```python
from build123d import *

# Parameters (mm, degrees)
SKETCH1_W           = 140
SKETCH1_H           = 60
SKETCH1_R           = 2.0955
BOSS_EXTRUDE1_DEPTH = 6.35
SKETCH2_W           = 16
SKETCH2_H           = 10
SKETCH2_R           = 2
BOSS_EXTRUDE2_DEPTH = 6.35
FILLET1_R           = 2


with BuildPart() as part:
    # Sketch1 → Boss-Extrude1 (new body)
    with BuildSketch(Plane.XZ):
        with Locations((-8.25, 0)):
            Rectangle(SKETCH1_W, SKETCH1_H)
        with Locations(Location((-73.25, 25, 0), (0, 0, 270))):
            Circle(SKETCH1_R, mode=Mode.SUBTRACT)
        with Locations(Location((0, 25, 0), (0, 0, 270))):
            Circle(SKETCH1_R, mode=Mode.SUBTRACT)
        with Locations(Location((56.75, 25, 0), (0, 0, 270))):
            Circle(SKETCH1_R, mode=Mode.SUBTRACT)
        with Locations(Location((56.75, -25, 0), (0, 0, 270))):
            Circle(SKETCH1_R, mode=Mode.SUBTRACT)
        with Locations(Location((0, -25, 0), (0, 0, 270))):
            Circle(SKETCH1_R, mode=Mode.SUBTRACT)
        with Locations(Location((-73.25, -25, 0), (0, 0, 270))):
            Circle(SKETCH1_R, mode=Mode.SUBTRACT)
    extrude(amount=BOSS_EXTRUDE1_DEPTH)

    # Sketch2 → Boss-Extrude2 (add)
    # profile 1 of 2: a face of its own
    with BuildSketch(Plane.XZ.offset(6.35)):
        with Locations((34.7, -35)):
            Rectangle(SKETCH2_W, SKETCH2_H)
        with Locations(Location((34.7, -35, 0), (0, 0, 270))):
            Circle(SKETCH2_R, mode=Mode.SUBTRACT)
    # profile 2 of 2: a face of its own
    with BuildSketch(Plane.XZ.offset(6.35)):
        with Locations((-51.2, 35)):
            Rectangle(SKETCH2_W, SKETCH2_H)
        with Locations(Location((-51.2, 35, 0), (0, 0, 270))):
            Circle(SKETCH2_R, mode=Mode.SUBTRACT)
    extrude(amount=-BOSS_EXTRUDE2_DEPTH)

    # Fillet1
    fillet1_edges = [part.edges().sort_by_distance(p)[0] for p in [
        (42.7, -3.175, -40),
        (26.7, -3.175, -40),
        (-59.2, -3.175, 40),
        (-43.2, -3.175, 40),
    ]]
    fillet(fillet1_edges, radius=FILLET1_R)


solid = part.part
```
Here's how the part is built. I have some questions about the finished solid (model axes, mm). A direction names the side the tool comes from. Coordinates: 2 decimals unless noted, no trailing zeros. Loops run counter-clockwise (first coordinate to the right, second up) from the corner with the lowest first, then second, coordinate; pieces in that order, holes last. Notation, with made-up numbers: (3, 70.5) - (39, 70.5) arc R23 cw to (39, 101.5) - close; hole circle Ø4 at (-39.5, 66.5). An arc over 180 degrees is marked (long way). Return JSON: item names as keys, results as strings. Group by question number.
Item 1: If we section it at A-A on z = 25: Write out the boundary of the cut face in (x, y).
Item 2: We'd pull the mould along X, two halves only. Please class faces 4 (the face through (-71.483, -3.131, -26.127)), 5 (the face through (-51, -3, 40)), 6 (the face through (26.7, -3, -34)): +X half, -X half, draft (parallel to the pull), parting line (faces both ways), or undercut.
Item 3: If we section it at C-C on x = 34.7: Write out the boundary of the cut face in (y, z).
Item 4: I need wall thicknesses on line 1 (X direction, y = -3.75, z = -25); line 2 (Z direction, x = -71.5, y = -3); line 3 (Z direction, x = -1, y = -4). Which ranges of each line are inside material? Lowest first, please. Write a range as from..to.
Item 5: If we section it at B-B on x = 56.75: Write out the boundary of the cut face in (y, z).
Item 6: On a 3-axis mill with a long thin cutter (end or side, diameter ignored), from which of +Z, -Z, +X, -X, +Y, -Y can I reach the whole of each face in a straight line? I mean faces 1 (the face through (-43.2, -3, 34)), 2 (the face through (52, -3, -30)), 3 (the face through (-27, -3, -30)). Say none if no direction works.
Item 7: Will these pins go through, and if not, where does the flat tip stop? P1, Ø2.5, axis at x = 56.75, z = 25, coming from the +Y side; P2, Ø5, axis at x = 0, z = -25, coming from the +Y side; P3, Ø3, axis at y = -1.5, z = 32.5, coming from the -X side; P4, Ø1.9, axis at x = 52, y = -2.5, coming from the -Z side.
Item 8: If we section it at D-D on y = -2.5: State how many separate pieces and enclosed holes the cut face has, and give its area (3 significant figures).
Calculated:
{
 "1": {"outline": "(-78.25, -6.35) - (-75.35, -6.35) - (-75.35, 0) - (-78.25, 0) - close; (-71.15, -6.35) - (-2.1, -6.35) - (-2.1, 0) - (-71.15, 0) - close; (2.1, -6.35) - (54.65, -6.35) - (54.65, 0) - (2.1, 0) - close; (58.85, -6.35) - (61.75, -6.35) - (61.75, 0) - (58.85, 0) - close"},
 "2": {"face 4": "undercut", "face 5": "draft", "face 6": "-X half"},
 "3": {"outline": "(-6.35, -40) - (0, -40) - (0, -37) - (-6.35, -37) - close; (-6.35, -33) - (0, -33) - (0, 30) - (-6.35, 30) - close"},
 "4": {"line 1": "x = -78.25..-75.35, -71.15..-2.1, 2.1..54.65, 58.85..61.75", "line 2": "z = -30..-26.15, -23.85..23.85, 26.15..30", "line 3": "z = -30..-26.84, -23.16..23.16, 26.84..30"},
 "5": {"outline": "(-6.35, -30) - (0, -30) - (0, -27.1) - (-6.35, -27.1) - close; (-6.35, -22.9) - (0, -22.9) - (0, 22.9) - (-6.35, 22.9) - close; (-6.35, 27.1) - (0, 27.1) - (0, 30) - (-6.35, 30) - close"},
 "6": {"face 1": "+Z, +X, +Y, -Y", "face 2": "-Z, +X, +Y, -Y", "face 3": "-Z, -X, +Y, -Y"},
 "7": {"P1": "passes through", "P2": "stops at y = 0", "P3": "stops at x = -59.2", "P4": "stops at z = -30"},
 "8": {"separate pieces": "1", "enclosed holes": "8", "area": "8,610 mm^2"}
}
